Geometry: final body of the model. Coordinates: model frame, mm. A direction names the side the tool comes from. Round coordinates to 2 decimals unless told otherwise and drop trailing zeros. Loops run counter-clockwise (first coordinate to the right, second up) from the corner with the lowest first, then second, coordinate; pieces in that order, holes last. Notation, with made-up numbers: M 45.5,-30 L 69.5,-30 A27 ccw 69.5,-14 Z; hole C 0,33 d6. An arc over 180 degrees is marked long. Answer as a JSON object with one key per item and string values.
from build123d import *

# Parameters (mm, degrees)
SKETCH2_W           = 6
SKETCH2_H           = 26.95
BOSS_EXTRUDE1_DEPTH = 9.6
CUT_EXTRUDE2_DEPTH  = 9.6
SKETCH7_W           = 1.5
SKETCH7_H           = 0.25
BOSS_EXTRUDE2_DEPTH = 9.6
SKETCH8_W           = 1.5
SKETCH8_H           = 3.25
BOSS_EXTRUDE3_DEPTH = 9.6


with BuildPart() as part:
    # Sketch2 → Boss-Extrude1 (new body)
    with BuildSketch(Plane(origin=(0, 0, 0), x_dir=(1, 0, 0), z_dir=(0, 1, 0))):
        with Locations((3, 13.475)):
            Rectangle(SKETCH2_W, SKETCH2_H)
    extrude(amount=BOSS_EXTRUDE1_DEPTH)

    # Sketch3 → Cut-Extrude2 (cut)
    with BuildSketch(Plane(origin=(0, 9.6, 0), x_dir=(1, 0, 0), z_dir=(0, 1, 0))):
        Polygon((3, 26.95), (2.25, 26.95), (2.25, 0), (3.75, 0), (3.75, 26.95), align=None)
    extrude(amount=-CUT_EXTRUDE2_DEPTH, mode=Mode.SUBTRACT)


with BuildPart() as cut_extrude2_piece_1:
    # of the separate pieces the step leaves, piece 1, a body of its own (cut_extrude2_pieces)
    add(part.part.solids().sort_by_distance((6, 0, 0))[0])



with BuildPart() as cut_extrude2_piece_2:
    # of the separate pieces the step leaves, piece 2, a body of its own (cut_extrude2_pieces)
    add(part.part.solids().sort_by_distance((0, 0, 0))[0])


with BuildPart() as cut_extrude2_piece_1_1:
    add(cut_extrude2_piece_1.part)

    add(cut_extrude2_piece_2.part)  # Boss-Extrude2 merges Cut-Extrude2 piece 2
    # Sketch7 → Boss-Extrude2 (add)
    with BuildSketch(Plane(origin=(0, 9.6, 0), x_dir=(1, 0, 0), z_dir=(0, 1, 0))):
        with Locations((3, 0.125)):
            Rectangle(SKETCH7_W, SKETCH7_H)
    extrude(amount=-BOSS_EXTRUDE2_DEPTH)

    # Sketch8 → Boss-Extrude3 (add)
    with BuildSketch(Plane(origin=(0, 9.6, 0), x_dir=(1, 0, 0), z_dir=(0, 1, 0))):
        with Locations((3, 25.325)):
            Rectangle(SKETCH8_W, SKETCH8_H)
    extrude(amount=-BOSS_EXTRUDE3_DEPTH)


solid = cut_extrude2_piece_1_1.part
1) Section query B-B (x = 2.95). Return the cut outline in (y, z), and give its area (3 significant figures).
Results:
{"outline": "M 0,-26.95 L 9.6,-26.95 L 9.6,-23.7 L 0,-23.7 Z; M 0,-0.25 L 9.6,-0.25 L 9.6,0 L 0,0 Z", "area": "33.6 mm2"}
2) Section query A-A (z = -4.5). Return the cut outline in (x, y).
Results:
{"outline": "M 0,0 L 2.25,0 L 2.25,9.6 L 0,9.6 Z; M 3.75,0 L 6,0 L 6,9.6 L 3.75,9.6 Z"}
3) Reachability of faces 1 (the flat face through (0, 5, -13)), 2 (the flat face through (3.75, 5, -12)) from +Z, -Z, +X, -X, +Y, -Y: full face, straight path, thin tool, end or side. Return the list, or none.
Results:
{"face 1": "+Z, -Z, -X, +Y, -Y", "face 2": "+Y, -Y"}
4) Section query C-C (y = 4.25). Return the cut outline in (x, z).
Results:
{"outline": "M 0,-26.95 L 6,-26.95 L 6,0 L 0,0 Z; hole M 2.25,-23.7 L 3.75,-23.7 L 3.75,-0.25 L 2.25,-0.25 Z"}
5) Ray query, line 1 (X direction, y = 2.5, z = -23.5); line 2 (Z direction, x = 2.95, y = 2.75). Return the intervals inside material, ascending.
Results:
{"line 1": "0 to 2.25, 3.75 to 6", "line 2": "-26.95 to -23.7, -0.25 to 0"}
6) Pull-direction query (X, two-part tool) for faces 3 (the flat face through (2, 9.6, -14)), 4 (the flat face through (3, 5, -0.25)), 5 (the flat face through (3, 5, -23.7)), 6 (the flat face through (6, 5, -13)); classes: +X half, -X half, draft (parallel to the pull), parting line (faces both ways), or undercut.
Results:
{"face 3": "draft", "face 4": "undercut", "face 5": "undercut", "face 6": "+X half"}
